Source: CAD feature listing. Evaluate the final solid. Frame: model axes, mm. A direction names the side the tool comes from. Coordinates: 2 decimals unless noted, no trailing zeros. Loops run counter-clockwise (first coordinate to the right, second up) from the corner with the lowest first, then second, coordinate; pieces in that order, holes last. Notation, with made-up numbers: M 68,78.5 L 126,78.5 A29 cw 126,107.5 Z; hole C -14,21.25 d11. An arc over 180 degrees is marked long. Write each question's results on one line, items separated by ' | '. Start each with the question number.
from build123d import *

# Parameters (mm, degrees)
SKETCH1_R                = 3.937
BOSS_EXTRUDE1_DEPTH      = 25.4
SKETCH2_W                = 1.905
SKETCH2_H                = 1.2192
BOSS_EXTRUDE2_DEPTH      = 25.4
FILLET2_R                = 0.254
CIRPATTERN4_COUNT        = 7
FILLET2_OF_CIRPATTERN4_R = 0.254
SKETCH3_R                = 3.048
CUT_EXTRUDE1_DEPTH       = 27.387619956


with BuildPart() as part:
    # Sketch1 → Boss-Extrude1 (new body)
    with BuildSketch(Plane(origin=(0, 0, 0), x_dir=(1, 0, 0), z_dir=(0, 1, 0))):
        with Locations(Location((0, 0, 0), (0, 0, 270))):
            Circle(SKETCH1_R)
    extrude(amount=BOSS_EXTRUDE1_DEPTH)

    # Sketch2 → Boss-Extrude2 (add)
    with BuildSketch(Plane(origin=(0, 25.4, 0), x_dir=(1, 0, 0), z_dir=(0, 1, 0))):
        with Locations((0, 4.429640936)):
            Rectangle(SKETCH2_W, SKETCH2_H)
    boss_extrude2 = extrude(amount=-BOSS_EXTRUDE2_DEPTH)

    # Fillet2
    fillet2_edges = [part.edges().sort_by_distance(p)[0] for p in [
        (0.9525, 12.7, -5.039240936),
        (0.9525, 12.7, -3.820040936),
        (-0.9525, 12.7, -3.820040936),
        (-0.9525, 12.7, -5.039240936),
    ]]
    fillet(fillet2_edges, radius=FILLET2_R)

    # CirPattern4: Boss-Extrude2 ×7 about axis
    cirpattern4_axis = Axis((0, 0, 0), (0, 1, 0))
    for i in range(1, CIRPATTERN4_COUNT):
        add(boss_extrude2.rotate(cirpattern4_axis, i * 360 / CIRPATTERN4_COUNT))

    # Fillet2 of CirPattern4
    fillet2_of_cirpattern4_edges = [part.edges().sort_by_distance(p)[0] for p in [
        (-3.345963175, 12.7, -3.88660982),
        (-2.392754232, 12.7, -3.126451053),
        (-3.580502304, 12.7, -1.637062079),
        (-4.533711247, 12.7, -2.397220845),
        (-5.124847834, 12.7, 0.192717763),
        (-3.936215723, 12.7, -0.07857976),
        (-3.512313344, 12.7, 1.778657913),
        (-4.700945455, 12.7, 2.049955436),
        (-3.044617546, 12.7, 4.126924939),
        (-2.515626491, 12.7, 3.028463696),
        (-0.799280798, 12.7, 3.855012219),
        (-1.328271853, 12.7, 4.953473462),
        (1.328271853, 12.7, 4.953473462),
        (0.799280798, 12.7, 3.855012219),
        (2.515626491, 12.7, 3.028463696),
        (3.044617546, 12.7, 4.126924939),
        (4.700945455, 12.7, 2.049955436),
        (3.512313344, 12.7, 1.778657913),
        (3.936215723, 12.7, -0.07857976),
        (5.124847834, 12.7, 0.192717763),
        (4.533711247, 12.7, -2.397220845),
        (3.580502304, 12.7, -1.637062079),
        (2.392754232, 12.7, -3.126451053),
        (3.345963175, 12.7, -3.88660982),
    ]]
    fillet(fillet2_of_cirpattern4_edges, radius=FILLET2_OF_CIRPATTERN4_R)

    # Sketch3 → Cut-Extrude1 (cut, through all)
    with BuildSketch(Plane(origin=(0, 25.4, 0), x_dir=(1, 0, 0), z_dir=(0, 1, 0))):
        with Locations(Location((0, 0, 0), (0, 0, 270))):
            Circle(SKETCH3_R)
    extrude(amount=-CUT_EXTRUDE1_DEPTH, mode=Mode.SUBTRACT)


solid = part.part
Item 1: First-contact query: pin 1 Ø1 at (x, y) = (2.5, 6) entering from +Z; pin 2 Ø4 at (y, z) = (12, 2) entering from -X; pin 3 Ø0.6 at (y, z) = (13.5, -4.5) entering from +X. Flat tips, straight axial feed; report the tip coordinate or a pass-through.
Item 2: Line query: probe 1 along X at (y, z) = (5.5, -3.5); probe 2 along Z at (x, y) = (0.5, 21); probe 3 along Z at (x, y) = (1.5, 11.25). Output: solid intervals per line, ascending.
Item 3: Mould query, pull axis X, two halves, no side actions, for faces 1 (the cylindrical face through (-3.836, 12.522, -0.884)), 2 (the cylindrical face through (-1.7, 12.52, -3.55)), 3 (the flat face through (0, 13, -5.039)), 4 (the flat face through (2.195, 12.878, 4.536)). Classes: +X half, -X half, draft (parallel to the pull), parting line (faces both ways), or undercut.
Item 4: Cut plane A-A (x = 0). Output: boundary loops of the cut face in (y, z).
Item 5: Cut plane B-B (z = -0.5). Output: boundary loops of the cut face in (x, y), then the cut area to 3 significant figures.
Item 6: Access query for faces 5 (the flat face through (-2.178, 12.878, 4.544)), 6 (the cylindrical face through (1.72, 12.52, -3.54)), 7 (the cylindrical face through (3.84, 12.52, -0.87)). Directions: +Z, -Z, +X, -X, +Y, -Y. A direction counts if a zero-diameter tool reaches every point of the face in a straight line with its end or side. Return the directions, or none.
Response values:
1) pin 1: stops at z = 4.63 | pin 2: stops at x = -5.07 | pin 3: stops at x = 0.95
2) probe 1: x = -3.65 to -2.86, -1.8 to 1.8, 2.86 to 3.65 | probe 2: z = -5.04 to -3.01, 3.01 to 3.91 | probe 3: z = -3.64 to -2.65, 2.65 to 4.86
3) face 1: -X half | face 2: undercut | face 3: draft | face 4: +X half
4) outline: M 0,-5.04 L 25.4,-5.04 L 25.4,-3.05 L 0,-3.05 Z; M 0,3.05 L 25.4,3.05 L 25.4,3.94 L 0,3.94 Z
5) outline: M -3.91,0 L -3.01,0 L -3.01,25.4 L -3.91,25.4 Z; M 3.01,0 L 3.91,0 L 3.91,25.4 L 3.01,25.4 Z | area: 45.6 mm2
6) face 5: +Z, -X, +Y, -Y | face 6: -Z, +Y, -Y | face 7: +X, +Y, -Y
